Input: part model. Units: mm. Frame: model coordinates. Face numbers are marked on the shaded views. A direction names the side the tool comes from. Coordinates: 2 decimals unless noted, no trailing zeros. Order: outer loops, then holes, each group sorted by start corner. A loop starts at its lowest first (then second) coordinate and runs counter-clockwise, first axis right, second up. Notation, with made-up numbers: (87, 58.25) -> (137, 58.25) arc R28 cw to (137, 88.25) -> close; hole circle Ø7 at (53, -19.75). An arc over 180 degrees is marked (long way). Use one line per item in the form item = value. Start each with the question number.
1) Ray query, line 1 along Y through (x, z) = (-3, 0); line 2 along X through (y, z) = (24.13, 11.5); line 3 along Z through (x, y) = (14, 18.5). Return the intervals inside material, ascending.
2) Section query D-D on y = 34. Output: boundary loops of the cut face in (x, z), then the cut area to 3 significant figures.
3) Section query A-A on x = 0. Count the separate pieces of the cut face and the enclosed holes in it, then the cut area to 3 significant figures.
4) Pin query (flat end, axial travel): pin 1 (6 mm diameter, centred on x = 3, z = 3.5, fed in from -Y); pin 2 (12 mm diameter, centred on x = -10, y = 23, fed in from -Z); pin 3 (6 mm diameter, centred on x = 13, y = 13.5, fed in from -Z); pin 4 (1.9 mm diameter, centred on x = 0, y = 24.13, fed in from +Z). Return the tip coordinate at first contact, or that it passes through.
5) Access query for the marked faces 1 and 2. Directions: +Z, -Z, +X, -X, +Y, -Y. A direction counts if a zero-diameter tool reaches every point of the face in a straight line with its end or side. Return the directions, or none.
6) Section query B-B on y = 24.13. Output: boundary loops of the cut face in (x, z).
from build123d import *

# Parameters (mm, degrees)
SKETCH1_W           = 38.862
SKETCH1_H           = 25.4
BOSS_EXTRUDE1_DEPTH = 17.78
SKETCH2_R           = 1.5875
CUT_EXTRUDE1_DEPTH  = 45.583331459
CUT_EXTRUDE2_DEPTH  = 45.583331459
SKETCH4_W           = 38.862
SKETCH4_H           = 25.4
BOSS_EXTRUDE2_DEPTH = 5.08
SKETCH5_R           = 1.5875
CUT_EXTRUDE3_DEPTH  = 25.4
CUT_EXTRUDE4_DEPTH  = 56.027210941
CUT_EXTRUDE5_DEPTH  = 56.027210941


with BuildPart() as part:
    # Sketch1 → Boss-Extrude1 (new body)
    with BuildSketch(Plane(origin=(0, 0, 0), x_dir=(1, 0, 0), z_dir=(0, 1, 0))):
        Rectangle(SKETCH1_W, SKETCH1_H)
    extrude(amount=BOSS_EXTRUDE1_DEPTH)

    # Sketch2 → Cut-Extrude1 (cut, through all)
    with BuildSketch(Plane(origin=(19.431, 0, 0), x_dir=(0, 0, -1), z_dir=(1, 0, 0))):
        with Locations((0, 6.35)):
            Circle(SKETCH2_R)
    extrude(amount=-CUT_EXTRUDE1_DEPTH, mode=Mode.SUBTRACT)

    # Sketch3 → Cut-Extrude2 (cut, through all)
    with BuildSketch(Plane(origin=(19.431, 0, 0), x_dir=(0, 0, -1), z_dir=(1, 0, 0))):
        with BuildLine():
            Line((-7.62, 17.78), (-7.62, 11.43))
            ThreePointArc((-7.62, 11.43), (-6.876051224, 9.633948776), (-5.08, 8.89))
            Line((-5.08, 8.89), (0, 8.89))
            ThreePointArc((0, 8.89), (1.796051224, 8.146051224), (2.54, 6.35))
            Line((2.54, 6.35), (2.54, 0))
            Line((2.54, 0), (12.7, 0))
            Line((12.7, 0), (12.7, 17.78))
            Line((12.7, 17.78), (-7.62, 17.78))
        make_face()
    extrude(amount=-CUT_EXTRUDE2_DEPTH, mode=Mode.SUBTRACT)

    # Sketch4 → Boss-Extrude2 (add)
    with BuildSketch(Plane(origin=(0, 0, 7.62), x_dir=(-1, 0, 0), z_dir=(0, 0, -1))):
        with Locations((0, 24.13)):
            Rectangle(SKETCH4_W, SKETCH4_H)
    extrude(amount=-BOSS_EXTRUDE2_DEPTH)

    # Sketch5 → Cut-Extrude3 (cut)
    with BuildSketch(Plane(origin=(0, 0, 7.62), x_dir=(-1, 0, 0), z_dir=(0, 0, -1))):
        with Locations(Location((0, 24.13, 0), (0, 0, 90))):
            Circle(SKETCH5_R)
    extrude(amount=-CUT_EXTRUDE3_DEPTH, mode=Mode.SUBTRACT)

    # Sketch6 → Cut-Extrude4 (cut, through all)
    with BuildSketch(Plane(origin=(19.431, 0, 0), x_dir=(0, 0, -1), z_dir=(1, 0, 0))):
        with BuildLine():
            ThreePointArc((2.1e-08, 0), (-2.046508636, 0.338818552), (-3.874625133, 1.319117366))
            Line((-3.874625133, 1.319117366), (-12.7, 8.116139232))
            Line((-12.7, 8.116139232), (-12.7, 0))
            Line((-12.7, 0), (2.1e-08, 0))
        make_face()
        with BuildLine():
            ThreePointArc((2.54, 0.530128867), (1.297366248, 0.133944915), (2.1e-08, 0))
            Line((2.1e-08, 0), (2.54, 0))
            Line((2.54, 0), (2.54, 0.530128867))
        make_face()
    extrude(amount=-CUT_EXTRUDE4_DEPTH, mode=Mode.SUBTRACT)

    # Sketch7 → Cut-Extrude5 (cut, through all)
    with BuildSketch(Plane(origin=(19.431, 0, 0), x_dir=(0, 0, -1), z_dir=(1, 0, 0))):
        with BuildLine():
            Line((-12.7, 8.436739039), (-3.719640128, 1.520352671))
            ThreePointArc((-3.719640128, 1.520352671), (-0.688923818, 0.293053577), (2.54, 0.808374246))
            Line((2.54, 0.808374246), (2.54, 0.530128867))
            ThreePointArc((2.54, 0.530128867), (-0.775197894, 0.047495083), (-3.874625133, 1.319117366))
            Line((-3.874625133, 1.319117366), (-12.7, 8.116139232))
            Line((-12.7, 8.116139232), (-12.7, 8.436739039))
        make_face()
    extrude(amount=-CUT_EXTRUDE5_DEPTH, mode=Mode.SUBTRACT)


solid = part.part
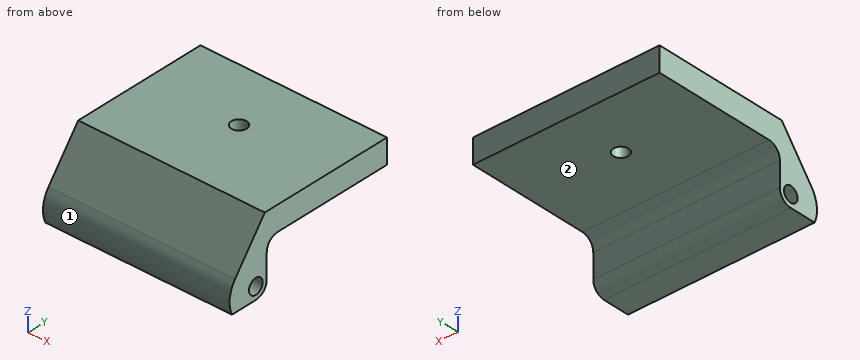
Answers below:
q1.line_1 = 0.25 to 4.76, 7.94 to 8.89
q1.line_2 = -19.43 to -1.59, 1.59 to 19.43
q1.line_3 = 7.62 to 12.7
q2.outline = (-19.43, 7.62) -> (19.43, 7.62) -> (19.43, 12.7) -> (-19.43, 12.7) -> close
q2.area = 197 mm^2
q3.separate_pieces = 2
q3.enclosed_holes = 1
q3.area = 205 mm^2
q4.pin_1 = 0.27
q4.pin_2 = 7.62
q4.pin_3 = 7.44
q4.pin_4 = through
q5.face_1 = +X, -X, -Y
q5.face_2 = -Z, +X, -X, +Y
q6.outline = (-19.43, 7.62) -> (-1.59, 7.62) -> (-1.59, 12.7) -> (-19.43, 12.7) -> close; (1.59, 7.62) -> (19.43, 7.62) -> (19.43, 12.7) -> (1.59, 12.7) -> close
